For this review, use the dimensioned drawing (mm, ordinates from the lowest corner) and the shaded views. A direction names the side the tool comes from. Coordinates: 2 decimals unless noted, no trailing zeros. Write each loop counter-clockwise with the first axis right and the second up, starting at its lowest first coordinate (ties: lowest second). Pieces come first, ordered by that corner, then holes. Notation, with made-up numbers: (38.5, 34) - (46.5, 34) arc R30 ccw to (46.5, 73) - close; hole circle Ø8 at (86, 70.5). An arc over 180 degrees is marked (long way). Answer as a JSON object with one key per item and string values.
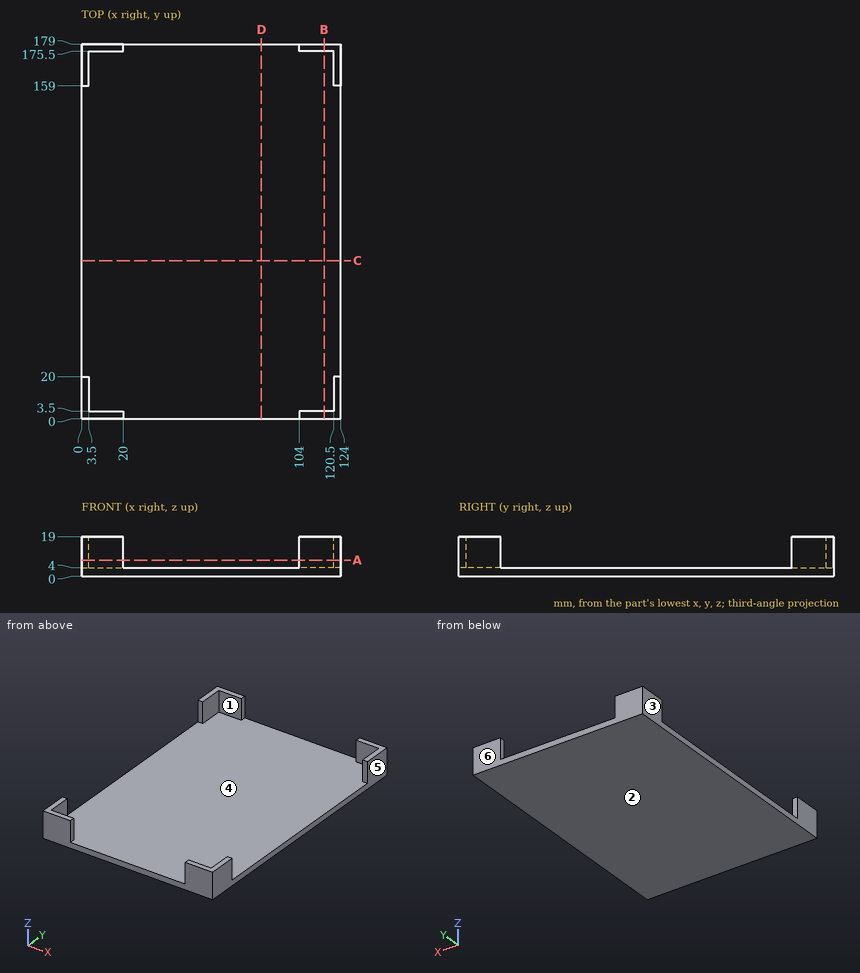
(1) Take a section at C-C, the plane y = 75.5. Write out the cut boundary in (x, z), and give its area (3 significant figures).
Solved:
{"outline": "(0, 0) - (124, 0) - (124, 4) - (0, 4) - close", "area": "496 mm^2"}
(2) Take a section at D-D, the plane x = 86. Write out the cut boundary in (y, z).
Solved:
{"outline": "(0, 0) - (179, 0) - (179, 4) - (0, 4) - close"}
(3) Tool access review of the marked faces 1 and 2: name each direction out of +Z, -Z, +X, -X, +Y, -Y from which nothing blocks a thin tool from reaching the whole face with its end or side.
Solved:
{"face 1": "+Z", "face 2": "-Z, +X, -X, +Y, -Y"}
(4) To check wall thickness, follow line 1 (Y direction, x = 10, z = 5.25); line 2 (X direction, y = 16.5, z = 9.25); line 3 (Z direction, x = 68.5, y = 28). State the ranges of each line that lie inside material, in increasing order. Write a range as from..to.
Solved:
{"line 1": "y = 0..3.5, 175.5..179", "line 2": "x = 0..3.5, 120.5..124", "line 3": "z = 0..4"}
(5) For pin 1 (1 mm diameter, centred on y = 178, z = 11, fed in from -X); pin 2 (12 mm diameter, centred on x = 102.5, y = 110.5, fed in from +Z), all flat-tipped, find the tip position at first contact; note any pin that passes through.
Solved:
{"pin 1": "stops at x = 0", "pin 2": "stops at z = 4"}
(6) Take a section at A-A, the plane z = 7.75. Write out the cut boundary in (x, y).
Solved:
{"outline": "(0, 0) - (20, 0) - (20, 3.5) - (3.5, 3.5) - (3.5, 20) - (0, 20) - close; (0, 159) - (3.5, 159) - (3.5, 175.5) - (20, 175.5) - (20, 179) - (0, 179) - close; (104, 0) - (124, 0) - (124, 20) - (120.5, 20) - (120.5, 3.5) - (104, 3.5) - close; (104, 175.5) - (120.5, 175.5) - (120.5, 159) - (124, 159) - (124, 179) - (104, 179) - close"}
(7) The part is to be moulded in two halves that separate along X. For the marked faces 3, 4, 5 and 6, say which applies: pulls with the +X half, pulls with the -X half, needs draft (parallel to the pull), parting line crosses it, or undercut.
Solved:
{"face 3": "pulls with the -X half", "face 4": "undercut", "face 5": "pulls with the +X half", "face 6": "needs draft"}
(8) Take a section at B-B, the plane x = 116. Write out the cut boundary in (y, z), and give its area (3 significant figures).
Solved:
{"outline": "(0, 0) - (179, 0) - (179, 19) - (175.5, 19) - (175.5, 4) - (3.5, 4) - (3.5, 19) - (0, 19) - close", "area": "821 mm^2"}
